```python
from build123d import *

# Parameters (mm, degrees)
SKETCH_1_W                                           = 34
SKETCH_1_H                                           = 41
EXTRUDE_1_DEPTH                                      = 5
FILLET_1_R                                           = 8
SKETCH_2_R                                           = 3
CUT_EXTRUDE_2_DEPTH                                  = 5
SKETCH_3_R                                           = 4
CUT_EXTRUDE_3_DEPTH                                  = 5
SKETCH_4_R                                           = 5
CUT_EXTRUDE_4_DEPTH                                  = 4
HOLE_WIZARD_M2_5_1_D                                 = 2.05
HOLE_WIZARD_M2_5_1_DEPTH                             = 7.35
HOLE_WIZARD_M2_5_1_TIP                               = 0.615882135
CUT_EXTRUDE_5_DEPTH                                  = 5
EXTRUDE1_DEPTH                                       = 5
SKETCH_8_R                                           = 1
CUT_EXTRUDE_6_DEPTH                                  = 5
CUT_EXTRUDE_7_DEPTH                                  = 2.5
SKETCH_10_R                                          = 3
CUT_EXTRUDE_8_DEPTH                                  = 1.8
CBORE_FOR_M2_5_HEXAGON_SOCKET_HEAD_CAP_S_D           = 2.7
CBORE_FOR_M2_5_HEXAGON_SOCKET_HEAD_CAP_S_CBORE_D     = 5
CBORE_FOR_M2_5_HEXAGON_SOCKET_HEAD_CAP_S_CBORE_DEPTH = 2.5
CBORE_FOR_M2_5_HEXAGON_SOCKET_HEAD_C_2_D             = 2.7
CBORE_FOR_M2_5_HEXAGON_SOCKET_HEAD_C_2_CBORE_D       = 5
CBORE_FOR_M2_5_HEXAGON_SOCKET_HEAD_C_2_CBORE_DEPTH   = 2.5
SKETCH_20_W                                          = 5
SKETCH_20_H                                          = 12
EXTRUDE_1_2_DEPTH                                    = 3
FILLET_2_R                                           = 1
M3X0_5_1_D                                           = 2.5
M3X0_5_1_CSINK_D                                     = 3.05
M3X0_5_1_CSINK_ANGLE                                 = 90


with BuildPart() as part:
    # 草图1 → Extrude 1 (new body)
    with BuildSketch(Plane.XY):
        with Locations((17, -20.5)):
            Rectangle(SKETCH_1_W, SKETCH_1_H)
    extrude(amount=EXTRUDE_1_DEPTH)

    # 圆角1
    fillet_1_edges = [part.edges().sort_by_distance(p)[0] for p in [
        (0, -41, 2.5),
    ]]
    fillet(fillet_1_edges, radius=FILLET_1_R)

    # 草图2 → 拉伸2 (cut)
    with BuildSketch(Plane.XY.offset(5)):
        with Locations((26, -35)):
            Circle(SKETCH_2_R)
    extrude(amount=-CUT_EXTRUDE_2_DEPTH, mode=Mode.SUBTRACT)

    # 草图3 → 拉伸3 (cut)
    with BuildSketch(Plane.XY.offset(5)):
        with Locations((5.5, -11)):
            Circle(SKETCH_3_R)
    extrude(amount=-CUT_EXTRUDE_3_DEPTH, mode=Mode.SUBTRACT)

    # 草图4 → 拉伸4 (cut)
    with BuildSketch(Plane.XY.offset(5)):
        with Locations((5.5, -11)):
            Circle(SKETCH_4_R)
    extrude(amount=-CUT_EXTRUDE_4_DEPTH, mode=Mode.SUBTRACT)

    # M2.5 螺纹孔1
    with Locations(Plane(origin=(3, 0, 2.5), x_dir=(0, 0, 1), z_dir=(0, 1, 0))):
        with Locations((0, 0), (0, 21)):
            Hole(HOLE_WIZARD_M2_5_1_D / 2, depth=HOLE_WIZARD_M2_5_1_DEPTH)
            with Locations((0, 0, -(HOLE_WIZARD_M2_5_1_DEPTH + HOLE_WIZARD_M2_5_1_TIP / 2))):  # 118° drill point
                Cone(0, HOLE_WIZARD_M2_5_1_D / 2, HOLE_WIZARD_M2_5_1_TIP, mode=Mode.SUBTRACT)

    # 草图7 → 拉伸5 (cut)
    with BuildSketch(Plane(origin=(0, 0, 0), x_dir=(-1, 0, 0), z_dir=(0, 0, -1))):
        with BuildLine():
            Line((-31.941608412, -34.164961394), (-27.140036221, 0))
            Line((-27.140036221, 0), (-34, 0))
            Line((-34, 0), (-34, -41))
            Line((-34, -41), (-26, -41))
            ThreePointArc((-26, -41), (-30.528257481, -38.936354174), (-31.941608412, -34.164961394))
        make_face()
    extrude(amount=-CUT_EXTRUDE_5_DEPTH, mode=Mode.SUBTRACT)

    # Sketch1 → Extrude1 (add)
    with BuildSketch(Plane(origin=(0, 0, 0), x_dir=(-1, 0, 0), z_dir=(0, 0, -1))):
        with BuildLine():
            Line((-26, -41), (-12, -41))
            ThreePointArc((-12, -41), (-3.514718626, -37.485281374), (0, -29))
            Line((0, -29), (0, -28.019790857))
            Line((0, -28.019790857), (-29.441458618, -39.914912266))
            ThreePointArc((-29.441458618, -39.914912266), (-27.804234797, -40.722301704), (-26, -41))
        make_face()
    extrude(amount=-EXTRUDE1_DEPTH)

    # 草图8 → 拉伸6 (cut)
    with BuildSketch(Plane(origin=(0, 0, 0), x_dir=(-1, 0, 0), z_dir=(0, 0, -1))):
        with Locations((-2.5, -28)):
            Circle(SKETCH_8_R)
    extrude(amount=-CUT_EXTRUDE_6_DEPTH, mode=Mode.SUBTRACT)

    # 草图9 → 拉伸7 (cut)
    with BuildSketch(Plane(origin=(0, 0, 0), x_dir=(-1, 0, 0), z_dir=(0, 0, -1))):
        with BuildLine():
            Line((-0.761170966, -30.758620396), (-4.707879973, -32.195104998))
            ThreePointArc((-4.707879973, -32.195104998), (-5.472518378, -32.161720164), (-5.989592737, -31.59743252))
            Line((-5.989592737, -31.59743252), (-8.452137769, -24.831645651))
            ThreePointArc((-8.452137769, -24.831645651), (-8.418752936, -24.067007246), (-7.854465292, -23.549932887))
            Line((-7.854465292, -23.549932887), (-3.907756285, -22.113448285))
            ThreePointArc((-3.907756285, -22.113448285), (-3.14311788, -22.146833118), (-2.626043521, -22.711120762))
            Line((-2.626043521, -22.711120762), (-0.163498489, -29.476907632))
            ThreePointArc((-0.163498489, -29.476907632), (-0.196883322, -30.241546037), (-0.761170966, -30.758620396))
        make_face()
    extrude(amount=-CUT_EXTRUDE_7_DEPTH, mode=Mode.SUBTRACT)

    # 草图10 → 拉伸8 (cut)
    with BuildSketch(Plane(origin=(0, 0, 2.5), x_dir=(-1, 0, 0), z_dir=(0, 0, -1))):
        with Locations((-4, -28)):
            Circle(SKETCH_10_R)
    extrude(amount=-CUT_EXTRUDE_8_DEPTH, mode=Mode.SUBTRACT)

    # CBORE for M2.5 Hexagon socket head cap s (through all)
    with Locations(Plane(origin=(4, -35, 5), x_dir=(1, 0, 0), z_dir=(0, 0, 1))):
        with Locations((0, 0)):
            CounterBoreHole(CBORE_FOR_M2_5_HEXAGON_SOCKET_HEAD_CAP_S_D / 2, CBORE_FOR_M2_5_HEXAGON_SOCKET_HEAD_CAP_S_CBORE_D / 2, CBORE_FOR_M2_5_HEXAGON_SOCKET_HEAD_CAP_S_CBORE_DEPTH)

    # CBORE for M2.5 Hexagon socket head c 2 (through all)
    with Locations(Plane(origin=(9.5, -30, 5), x_dir=(1, 0, 0), z_dir=(0, 0, 1))):
        with Locations((0, 0)):
            CounterBoreHole(CBORE_FOR_M2_5_HEXAGON_SOCKET_HEAD_C_2_D / 2, CBORE_FOR_M2_5_HEXAGON_SOCKET_HEAD_C_2_CBORE_D / 2, CBORE_FOR_M2_5_HEXAGON_SOCKET_HEAD_C_2_CBORE_DEPTH)

    # 草图20 → Extrude 1 2 (add)
    with BuildSketch(Plane.ZY):
        with Locations((2.5, -11)):
            Rectangle(SKETCH_20_W, SKETCH_20_H)
    extrude(amount=EXTRUDE_1_2_DEPTH)

    # 圆角2
    fillet_2_edges = [part.edges().sort_by_distance(p)[0] for p in [
        (0, -17, 2.5),
        (0, -5, 2.5),
        (-3, -17, 2.5),
        (-3, -5, 2.5),
    ]]
    fillet(fillet_2_edges, radius=FILLET_2_R)

    # M3x0.5 螺纹孔1 (through all)
    with Locations(Plane(origin=(7, -3, 0), x_dir=(-1, 0, 0), z_dir=(0, 0, -1))):
        with Locations((0, 0)):
            CounterSinkHole(M3X0_5_1_D / 2, M3X0_5_1_CSINK_D / 2, counter_sink_angle=M3X0_5_1_CSINK_ANGLE)


solid = part.part
```
CAD build for the part. Positions are in the model's coordinates, mm. A direction names the side the tool comes from. Round coordinates to 2 decimals unless told otherwise and drop trailing zeros. Order: outer loops, then holes, each group sorted by start corner. A loop starts at its lowest first (then second) coordinate and runs counter-clockwise, first axis right, second up. Notation, with made-up numbers: (-12, -16.75) - (-4, -16.75) arc R35 ccw to (-4, 20.25) - close; hole circle Ø1 at (-2.75, 40.25). An arc over 180 degrees is marked (long way). Answer as CSV lines item,"result". Start each with the question number.
1. Drill centre lines: L1, parallel to Y at x = 26, z = 2.15; L2, parallel to Y at x = 5, z = 4.1; L3, parallel to Y at x = 5.5, z = 0.25. Where is each one in solid material? Low to high. Write a range as [from, to].
2. Tool access for faces 1 (the face through (1.815, -7.621, 3.028)), 2 (the face through (8.423, -24.077, 1.232)), 3 (the face through (-1.5, -17, 2.5)), 4 (the face through (25.016, -3.726, 2.633)): list every direction of +Z, -Z, +X, -X, +Y, -Y with a clear straight run to the whole face (end or side of a thin tool).
3. Saw through at B-B, the plane y = -10.5. Write the cut outline in (x, z), and give its area (3 significant figures).
4. Saw through at C-C, the plane y = -35. Write the cut outline in (x, z), and give its area (3 significant figures).
5. Saw through at A-A, the plane y = -3. Write the cut outline in (x, z) (3 decimals).
6. Saw through at D-D, the plane y = -24. Write the cut outline in (x, z).
7. Pull direction Y, two halves, no side cores. Call faces 5 (the face through (17, -41, 2)), 6 (the face through (14, -20, 0)), 7 (the face through (5.909, -22.842, 1.232)): +Y half, -Y half, draft (parallel to the pull), parting line (faces both ways), or undercut.
8. Pin check, flat tips, straight feed: pin 1 (1.1 mm diameter, centred on x = -1.5, z = 1.5, fed in from +Y); pin 2 (3 mm diameter, centred on x = 6, z = 1.5, fed in from -Y); pin 3 (2.5 mm diameter, centred on x = 2.5, y = -28, fed in from -Z); pin 4 (2 mm diameter, centred on x = 4, y = -35, fed in from -Z). Stop position of each tip, or through.
Model answer:
1,L1,"y = [-41, -38], [-32, 0]"
1,L2,"y = [-40.42, -37.29], [-32.71, -30.83], [-25.17, -15.97], [-6.03, 0]"
1,L3,"y = [-40.6, -32.15], [-22.69, -15], [-7, 0]"
2,face 1,"+Z"
2,face 2,"-Z"
2,face 3,"+Z, -Z, -X, -Y"
2,face 4,"+Y"
3,outline,"(-3, 0) - (1.53, 0) - (1.53, 1) - (0.53, 1) - (0.53, 5) - (-3, 5) - close; (9.47, 0) - (28.62, 0) - (28.62, 5) - (10.47, 5) - (10.47, 1) - (9.47, 1) - close"
3,area,"110 mm²"
4,outline,"(0.25, 0) - (2.65, 0) - (2.65, 2.5) - (1.5, 2.5) - (1.5, 5) - (0.25, 5) - close; (5.35, 0) - (23, 0) - (23, 5) - (6.5, 5) - (6.5, 2.5) - (5.35, 2.5) - close; (29, 0) - (32, 0) - (32, 5) - (29, 5) - close"
4,area,"109 mm²"
5,outline,"(0, 0) - (5.475, 0) - (5.75, 0.275) - (5.75, 5) - (0, 5) - close; (8.25, 0.275) - (8.525, 0) - (27.562, 0) - (27.562, 5) - (8.25, 5) - close; hole circle Ø2.05 at (3, 2.5); hole circle Ø2.05 at (24, 2.5)"
6,outline,"(0, 0) - (2.16, 0) - (2.16, 2.5) - (8.38, 2.5) - (8.38, 0) - (30.51, 0) - (30.51, 5) - (0, 5) - close"
7,face 5,"-Y half"
7,face 6,"draft"
7,face 7,"undercut"
8,pin 1,"stops at y = -5"
8,pin 2,"stops at y = -40.98"
8,pin 3,"stops at z = 4.3"
8,pin 4,"passes through"
